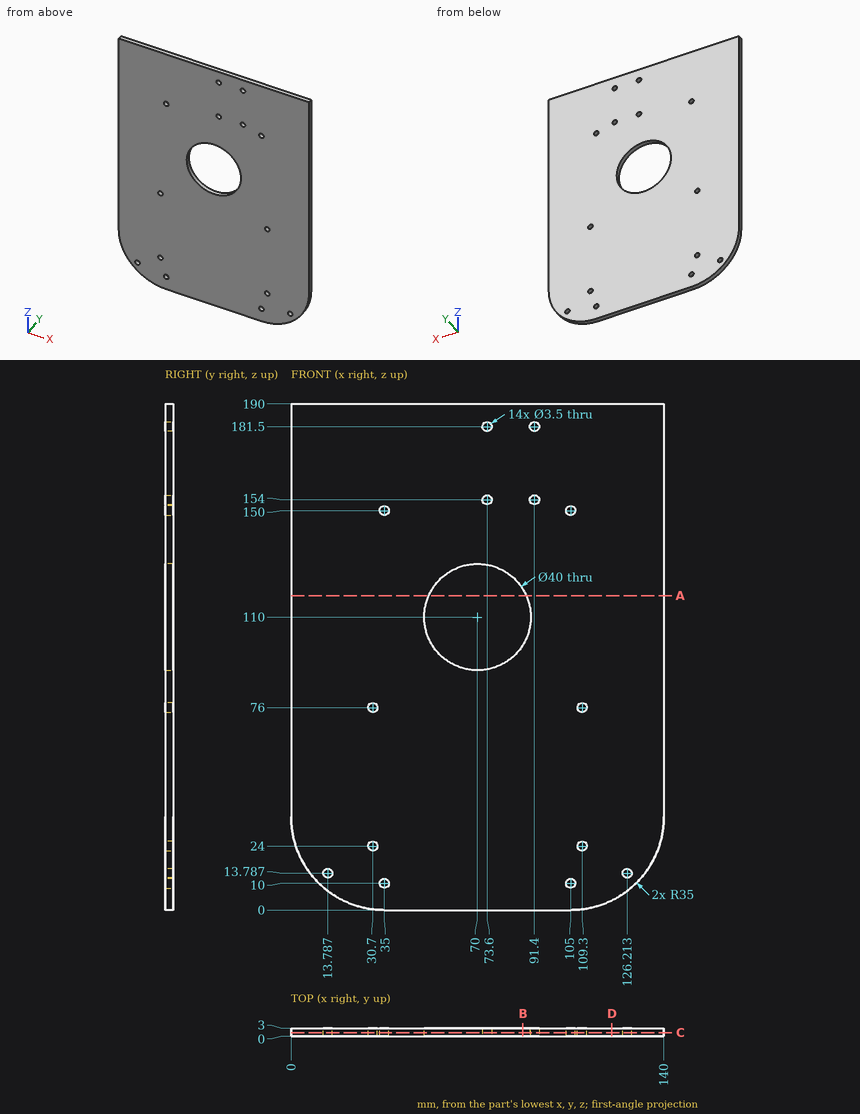
Verification items for this drawing (mm, ordinates from the low corner). Coordinates: 2 decimals unless noted, no trailing zeros. Write each loop counter-clockwise with the first axis right and the second up, starting at its lowest first coordinate (ties: lowest second). Pieces come first, ordered by that corner, then holes. Notation, with made-up numbers: M -33.75,-37 L 12.25,-37 A16 cw 12.25,-30 Z; hole C 29.25,17.25 d10. An arc over 180 degrees is marked long. Answer as CSV lines item,"result".
Q1. Cross-section at B-B (x = 87). Record the boundary of the cut face in (y, z).
Check result:
outline,"M 0,0 L 3,0 L 3,99.46 L 0,99.46 Z; M 0,120.54 L 3,120.54 L 3,190 L 0,190 Z"
Q2. Material ranges on probe 1 along X at (y, z) = (0.6, 76); probe 2 along X at (y, z) = (1.9, 154); probe 3 along Z at (x, y) = (91.4, 2.15), recorded low to high. Write a range as from..to.
Check result:
probe 1,"0..28.95, 32.45..107.55, 111.05..140"
probe 2,"0..71.85, 75.35..89.65, 93.15..140"
probe 3,"0..152.25, 155.75..179.75, 183.25..190"
Q3. Cross-section at A-A (z = 118). Record the boundary of the cut face in (x, y).
Check result:
outline,"M 0,0 L 51.67,0 L 51.67,3 L 0,3 Z; M 88.33,0 L 140,0 L 140,3 L 88.33,3 Z"
Q4. Cross-section at D-D (x = 120.5). Record the boundary of the cut face in (y, z), then the cut area to 3 significant figures.
Check result:
outline,"M 0,3.62 L 3,3.62 L 3,190 L 0,190 Z"
area,"559 mm^2"
Q5. Go/stop test with a flat-tipped pin: pin 1 (3 mm diameter, centred on x = 91.4, z = 181.5, fed in from +Y). Record where the tip stops, or that it passes through.
Check result:
pin 1,"through"
Q6. Cross-section at C-C (y = 1.3). Count the separate pieces of the cut face and the enclosed holes in it, then the cut area to 3 significant figures.
Check result:
separate pieces,"1"
enclosed holes,"15"
area,"24,700 mm^2"
